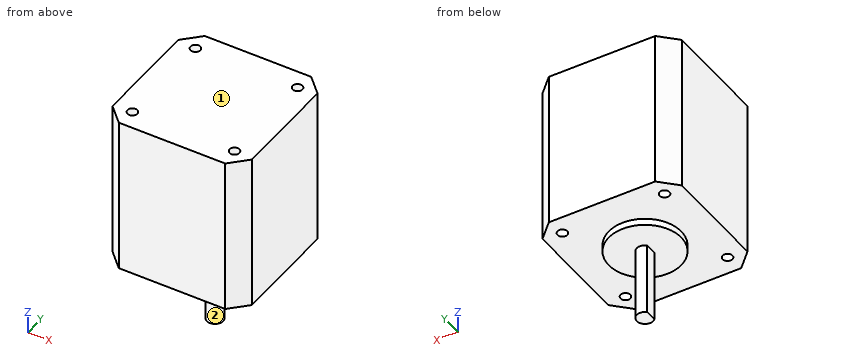
```python
from build123d import *

# Parameters (mm, degrees)
SKETCH1_R           = 1.5
BOSS_EXTRUDE1_DEPTH = 48
SKETCH1_5_R         = 11
BOSS_EXTRUDE2_DEPTH = 2
BOSS_EXTRUDE3_DEPTH = 24


with BuildPart() as part:
    # Sketch1 → Boss-Extrude1 (new body)
    with BuildSketch(Plane.XY):
        Polygon((-21.15, 16.15), (-16.15, 21.15), (16.15, 21.15), (21.15, 16.15), (21.15, -16.15), (16.15, -21.15), (-16.15, -21.15), (-21.15, -16.15), align=None)
        with Locations((-15.5, 15.5)):
            Circle(SKETCH1_R, mode=Mode.SUBTRACT)
        with Locations((-15.5, -15.5)):
            Circle(SKETCH1_R, mode=Mode.SUBTRACT)
        with Locations((15.5, -15.5)):
            Circle(SKETCH1_R, mode=Mode.SUBTRACT)
        with Locations((15.5, 15.5)):
            Circle(SKETCH1_R, mode=Mode.SUBTRACT)
    extrude(amount=BOSS_EXTRUDE1_DEPTH)

    # Sketch1<5> → Boss-Extrude2 (add)
    with BuildSketch(Plane.XY):
        Circle(SKETCH1_5_R)
    extrude(amount=-BOSS_EXTRUDE2_DEPTH)

    # Sketch1<6> → Boss-Extrude3 (add)
    with BuildSketch(Plane.XY):
        with BuildLine():
            Line((-1.767766953, 1.767766953), (-1.767766953, -1.767766953))
            ThreePointArc((-1.767766953, -1.767766953), (2.5, 0), (-1.767766953, 1.767766953))
        make_face()
    extrude(amount=-BOSS_EXTRUDE3_DEPTH)


solid = part.part
```
Build history of the part. All positions in model axes, mm. Face numbers are marked on the shaded views. A direction names the side the tool comes from. Coordinates: 2 decimals unless noted, no trailing zeros. Order: outer loops, then holes, each group sorted by start corner. A loop starts at its lowest first (then second) coordinate and runs counter-clockwise, first axis right, second up.
Item 1: Drill centre lines: L1, parallel to Y at x = 15.5, z = 37.5; L2, parallel to Z at x = 2.5, y = 17.5; L3, parallel to Y at x = -15, z = 29. Where is each one in solid material? Low to high.
Filled in:
L1: y = -21.15 to -17, -14 to 14, 17 to 21.15
L2: z = 0 to 48
L3: y = -21.15 to -16.91, -14.09 to 14.09, 16.91 to 21.15
Item 2: Tool access for the marked faces 1 and 2: list every direction of +Z, -Z, +X, -X, +Y, -Y with a clear straight run to the whole face (end or side of a thin tool).
Filled in:
face 1: +Z, +X, -X, +Y, -Y
face 2: -Z
Item 3: Saw through at A-A on z = 39.5. List the corners of the cut face in (x, y).
Filled in:
outline: (-21.15, -16.15) - (-16.15, -21.15) - (16.15, -21.15) - (21.15, -16.15) - (21.15, 16.15) - (16.15, 21.15) - (-16.15, 21.15) - (-21.15, 16.15) - close; hole circle Ø3 at (-15.5, -15.5); hole circle Ø3 at (-15.5, 15.5); hole circle Ø3 at (15.5, -15.5); hole circle Ø3 at (15.5, 15.5)
Item 4: Drop flat-ended pins along their axis: pin 1 Ø3.5 at (x, y) = (-15.5, 15.5) entering from -Z; pin 2 Ø1.1 at (y, z) = (-0.5, -12) entering from -X; pin 3 Ø1.8 at (x, y) = (-15.5, -15.5) entering from -Z; pin 4 Ø10 at (x, y) = (-13, 8.5) entering from -Z. Give the stop position or say it passes through.
Filled in:
pin 1: stops at z = 0
pin 2: stops at x = -1.77
pin 3: passes through
pin 4: stops at z = -2
Item 5: Saw through at D-D on z = -5. List the corners of the cut face in (x, y), then the cut area to 3 significant figures.
Filled in:
outline: (-1.77, -1.77) arc R2.5 ccw (long way) to (-1.77, 1.77) - close
area: 17.9 mm2
Item 6: Saw through at B-B on y = 0. List the corners of the cut face in (x, z), then the cut area to 3 significant figures.
Filled in:
outline: (-21.15, 0) - (-11, 0) - (-11, -2) - (-1.77, -2) - (-1.77, -24) - (2.5, -24) - (2.5, -2) - (11, -2) - (11, 0) - (21.15, 0) - (21.15, 48) - (-21.15, 48) - close
area: 2,170 mm2
Item 7: Saw through at C-C on x = -6. List the corners of the cut face in (y, z).
Filled in:
outline: (-21.15, 0) - (-9.22, 0) - (-9.22, -2) - (9.22, -2) - (9.22, 0) - (21.15, 0) - (21.15, 48) - (-21.15, 48) - close
